from build123d import *

# Parameters (mm, degrees)
SKETCH1_W           = 140.9
SKETCH1_H           = 54.3
SKETCH1_W_2         = 125.9
SKETCH1_H_2         = 39.3
BOSS_EXTRUDE1_DEPTH = 7.5
SKETCH2_W           = 7.5
SKETCH2_H           = 7.5
BOSS_EXTRUDE2_DEPTH = 75


with BuildPart() as part:
    # Sketch1 → Boss-Extrude1 (new body)
    with BuildSketch(Plane(origin=(0, 0, 0), x_dir=(1, 0, 0), z_dir=(0, 1, 0))):
        Rectangle(SKETCH1_W, SKETCH1_H)
        Rectangle(SKETCH1_W_2, SKETCH1_H_2, mode=Mode.SUBTRACT)
    extrude(amount=BOSS_EXTRUDE1_DEPTH)

    # Sketch2 → Boss-Extrude2 (add)
    with BuildSketch(Plane(origin=(0, 7.5, 0), x_dir=(1, 0, 0), z_dir=(0, 1, 0))):
        with Locations((-66.7, 23.4)):
            Rectangle(SKETCH2_W, SKETCH2_H)
        with Locations((66.7, 23.4)):
            Rectangle(SKETCH2_W, SKETCH2_H)
        with Locations((66.7, -23.4)):
            Rectangle(SKETCH2_W, SKETCH2_H)
        with Locations((-66.7, -23.4)):
            Rectangle(SKETCH2_W, SKETCH2_H)
    extrude(amount=BOSS_EXTRUDE2_DEPTH)


solid = part.part
Can you work these out from the model? Positions are in its coordinate system, mm. A direction names the side the tool comes from. Coordinates: 2 decimals unless noted, no trailing zeros. Loops run counter-clockwise (first coordinate to the right, second up) from the corner with the lowest first, then second, coordinate; pieces in that order, holes last. Notation, with made-up numbers: (24.25, 55) - (76.25, 55) arc R22 ccw to (76.25, 68) - close; hole circle Ø4 at (28.25, 41.5). An arc over 180 degrees is marked (long way). Answer as a JSON object with one key per item and string values. Group by question number.
Item 1: On a 3-axis mill with a long thin cutter (end or side, diameter ignored), from which of +Z, -Z, +X, -X, +Y, -Y can I reach the whole of each face in a straight line? I mean faces 1 (the face through (-62.95, 4, 0)), 2 (the face through (67, 44, -19.65)), 3 (the face through (62.95, 44, -23)). Say none if no direction works.
Item 2: If we section it at B-B (x = 15.5): List the corners of the cut face in (y, z) for me, plus the area to 4 significant figures.
Item 3: If I drill on L1, parallel to X at y = 14.5, z = 24; L2, parallel to Z at x = 64.5, y = 58.5; L3, parallel to Y at x = -5, z = 21, over which ranges is the centre line in solid material (lowest first)? Write a range as from..to.
Item 4: If we section it at C-C (z = -9): List the corners of the cut face in (x, y) for me, plus the area to 4 significant figures.
Item 5: If we section it at D-D (z = 24): List the corners of the cut face in (x, y) for me.
Item 6: For pin 1 (5 mm diameter, centred on x = -30.5, z = -21, fed in from +Y); pin 2 (2 mm diameter, centred on x = 7, z = -17, fed in from +Y), each with a flat end and sliding along its axis, tell me the tip position at first contact or that it passes through.
Item 7: If we section it at A-A (y = 16.5): List the corners of the cut face in (x, z) for me, plus the area to 3 significant figures.
Item 8: If we mould it in two halves opening along X, with no side actions, what happens to faces 4 (the face through (-1, 7.5, -23)), 5 (the face through (-70.45, 32, 20)), 6 (the face through (-67, 82.5, -23)), 7 (the face through (62.95, 4, 0))? For each: released by +X, released by -X, zero draft, split by the parting line, or undercut.
Returned:
{
 "1": {"face 1": "+Y, -Y", "face 2": "+X, -X, +Y", "face 3": "+Z, -Z, +Y"},
 "2": {"outline": "(0, -27.15) - (7.5, -27.15) - (7.5, -19.65) - (0, -19.65) - close; (0, 19.65) - (7.5, 19.65) - (7.5, 27.15) - (0, 27.15) - close", "area": "112.5 mm²"},
 "3": {"L1": "x = -70.45..-62.95, 62.95..70.45", "L2": "z = -27.15..-19.65, 19.65..27.15", "L3": "y = 0..7.5"},
 "4": {"outline": "(-70.45, 0) - (-62.95, 0) - (-62.95, 7.5) - (-70.45, 7.5) - close; (62.95, 0) - (70.45, 0) - (70.45, 7.5) - (62.95, 7.5) - close", "area": "112.5 mm²"},
 "5": {"outline": "(-70.45, 0) - (70.45, 0) - (70.45, 82.5) - (62.95, 82.5) - (62.95, 7.5) - (-62.95, 7.5) - (-62.95, 82.5) - (-70.45, 82.5) - close"},
 "6": {"pin 1": "stops at y = 7.5", "pin 2": "passes through"},
 "7": {"outline": "(-70.45, -27.15) - (-62.95, -27.15) - (-62.95, -19.65) - (-70.45, -19.65) - close; (-70.45, 19.65) - (-62.95, 19.65) - (-62.95, 27.15) - (-70.45, 27.15) - close; (62.95, -27.15) - (70.45, -27.15) - (70.45, -19.65) - (62.95, -19.65) - close; (62.95, 19.65) - (70.45, 19.65) - (70.45, 27.15) - (62.95, 27.15) - close", "area": "225 mm²"},
 "8": {"face 4": "undercut", "face 5": "released by -X", "face 6": "zero draft", "face 7": "undercut"}
}
